Here's how the part is built. I have some questions about the finished solid (model axes, mm). Face numbers are marked on the shaded views. Round coordinates to 2 decimals unless told otherwise and drop trailing zeros. Loops run counter-clockwise (first coordinate to the right, second up) from the corner with the lowest first, then second, coordinate; pieces in that order, holes last. Notation, with made-up numbers: (23, -17) - (51, -17) arc R37 ccw to (51, 22) - close; hole circle Ø7 at (25, 26.5). An arc over 180 degrees is marked (long way). Answer as a JSON object with one key per item and string values. Group by question number.
1) I want a section at D-D, the plane x = 0.8. Please give me the cut outline in (y, z), then the cut area to 3 significant figures.
2) I want a section at B-B, the plane y = 0.8. Please give me the cut outline in (x, z).
3) If I drill on line 1 along Z through (x, y) = (-0.7, -0.6); line 2 along Z through (x, y) = (1.75, 1); line 3 along Y through (x, z) = (0.65, 18), over which ranges is the centre line in solid material (lowest first)? Write a range as [from, to].
4) Will these pins go through, and if not, where does the flat tip stop? P1, Ø0.6, axis at y = -1, z = 14, coming from the -X side; P2, Ø1, axis at x = -1, y = -1.5, coming from the -Z side; P3, Ø1, axis at y = 1, z = 10, coming from the +X side.
5) I want a section at C-C, the plane z = 10.5. Please give me the cut outline in (x, y), then the cut area to 3 significant figures.
6) If we mould it in two halves opening along Z, with no side actions, what happens to the marked faces 1, 2, 3 and 4? For each: pulls with the +Z half, pulls with the -Z half, needs draft (parallel to the pull), parting line crosses it, or undercut.
7) I want a section at A-A, the plane x = -0.45. Please give me the cut outline in (y, z), then the cut area to 3 significant figures.
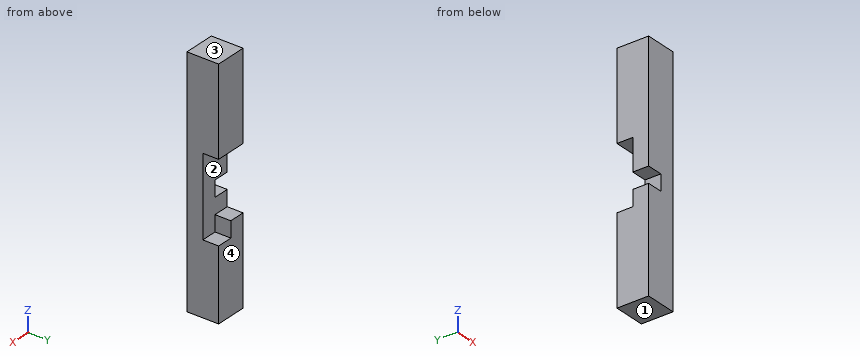
from build123d import *

# Parameters (mm, degrees)
SKETCH_1_W          = 4
SKETCH_1_H          = 4
EXTRUDE_1_DEPTH     = 30
SKETCH_4_W          = 10
SKETCH_4_H          = 2
CUT_EXTRUDE_1_DEPTH = 4
SKETCH_6_W          = 4
SKETCH_6_H          = 2
CUT_EXTRUDE_2_DEPTH = 2
SKETCH_8_W          = 2
SKETCH_8_H          = 2
EXTRUDE_4_DEPTH     = 2
SKETCH_10_W         = 2
SKETCH_10_H         = 2
EXTRUDE_6_DEPTH     = 2


with BuildPart() as part:
    # 草圖1 → 填料-伸長1 (new body)
    with BuildSketch(Plane.XY):
        Rectangle(SKETCH_1_W, SKETCH_1_H)
    extrude(amount=EXTRUDE_1_DEPTH)

    # 草圖4 → 除料-伸長1 (cut)
    with BuildSketch(Plane.ZY.offset(2)):
        with Locations((14, 1)):
            Rectangle(SKETCH_4_W, SKETCH_4_H)
    extrude(amount=-CUT_EXTRUDE_1_DEPTH, mode=Mode.SUBTRACT)

    # 草圖6 → 除料-伸長2 (cut)
    with BuildSketch(Plane.ZY.offset(2)):
        with Locations((13, -1)):
            Rectangle(SKETCH_6_W, SKETCH_6_H)
    extrude(amount=-CUT_EXTRUDE_2_DEPTH, mode=Mode.SUBTRACT)

    # 草圖8 → 填料-伸長4 (add)
    with BuildSketch(Plane.ZY.offset(2)):
        with Locations((10, 1)):
            Rectangle(SKETCH_8_W, SKETCH_8_H)
    extrude(amount=-EXTRUDE_4_DEPTH)

    # 草圖10 → 填料-伸長6 (add)
    with BuildSketch(Plane.XY.offset(11)):
        with Locations((-1, -1)):
            Rectangle(SKETCH_10_W, SKETCH_10_H)
    extrude(amount=EXTRUDE_6_DEPTH)


solid = part.part
Outcome:
{
 "1": {"outline": "(-2, 0) - (2, 0) - (2, 9) - (0, 9) - (0, 19) - (2, 19) - (2, 30) - (-2, 30) - close", "area": "100 mm^2"},
 "2": {"outline": "(-2, 0) - (2, 0) - (2, 9) - (0, 9) - (0, 11) - (-2, 11) - close; (-2, 19) - (2, 19) - (2, 30) - (-2, 30) - close"},
 "3": {"line 1": "[0, 13], [15, 30]", "line 2": "[0, 9], [19, 30]", "line 3": "[-2, 0]"},
 "4": {"P1": "x = 0", "P2": "z = 0", "P3": "x = 0"},
 "5": {"outline": "(-2, -2) - (2, -2) - (2, 0) - (0, 0) - (0, 2) - (-2, 2) - close", "area": "12.0 mm^2"},
 "6": {"face 1": "pulls with the -Z half", "face 2": "undercut", "face 3": "pulls with the +Z half", "face 4": "needs draft"},
 "7": {"outline": "(-2, 0) - (2, 0) - (2, 11) - (0, 11) - (0, 13) - (-2, 13) - close; (-2, 15) - (0, 15) - (0, 19) - (2, 19) - (2, 30) - (-2, 30) - close", "area": "100 mm^2"}
}
